```python
from build123d import *

# Parameters (mm, degrees)
SKETCH_1_W              = 20
SKETCH_1_H              = 25
EXTRUDE_1_DEPTH         = 1.5
SKETCH_2_W              = 10.1
SKETCH_2_H              = 17.5
CUT_EXTRUDE_1_DEPTH     = 0.25
HOLE_WIZARD_3_2_3_2_1_D = 3.2
HOLE_WIZARD_3_2_3_2_2_D = 3.2


with BuildPart() as part:
    # 草图1 → 凸台-拉伸1 (new body)
    with BuildSketch(Plane.XZ):
        with Locations((0, -2.5)):
            Rectangle(SKETCH_1_W, SKETCH_1_H)
    extrude(amount=-EXTRUDE_1_DEPTH)

    # 草图2 → 切除-拉伸1 (cut)
    with BuildSketch(Plane.XZ):
        with Locations((0, 1.25)):
            Rectangle(SKETCH_2_W, SKETCH_2_H)
    extrude(amount=-CUT_EXTRUDE_1_DEPTH, mode=Mode.SUBTRACT)

    # Ø3.2 (3.2) 直径孔1 (through all)
    with Locations(Plane(origin=(0, 0, 0), x_dir=(-1, 0, 0), z_dir=(0, -1, 0))):
        with Locations((-7, -7), (-7, 12)):
            Hole(HOLE_WIZARD_3_2_3_2_1_D / 2)

    # Ø3.2 (3.2) 直径孔2 (through all)
    with Locations(Plane(origin=(0, 1.5, 0), x_dir=(1, 0, 0), z_dir=(0, 1, 0))):
        with Locations((-7, -7), (-7, 12)):
            Hole(HOLE_WIZARD_3_2_3_2_2_D / 2)


solid = part.part
```
For this review, take the finished solid that the model builds, in its own axes (mm). A direction names the side the tool comes from. Coordinates: 2 decimals unless noted, no trailing zeros. Loops run counter-clockwise (first coordinate to the right, second up) from the corner with the lowest first, then second, coordinate; pieces in that order, holes last. Notation, with made-up numbers: (47, -40) - (91, -40) arc R25 ccw to (91, -26) - close; hole circle Ø8 at (1.25, -21.75). An arc over 180 degrees is marked (long way). Use one line per item in the form item = value. Start each with the question number.
1) To check wall thickness, follow probe 1 along X at (y, z) = (0.4, 7); probe 2 along Z at (x, y) = (-7, 0.7); probe 3 along Z at (x, y) = (7.5, 0.45). State the ranges of each line that lie inside material, in increasing order. Write a range as from..to.
2) Take a section at B-B (y = 0.8). State the section outline as (x, z) points.
3) Take a section at C-C (x = 7.25). State the section outline as (y, z) points.
4) Take a section at D-D (z = 2.75). State the section outline as (x, y) points.
5) For faces 4 (the face through (0, 1, 10)), 5 (the face through (0, 0.25, 1)), list the 3-axis set-ups (+Z, -Z, +X, -X, +Y, -Y) from which the entire face can be reached by the end or side of a thin tool; tool diameter is ignored.
6) Take a section at A-A (z = -12). State the section outline as (x, y) points.
7) For pin 1 (3 mm diameter, centred on x = -1.5, z = -0.5, fed in from -Y); pin 2 (3 mm diameter, centred on x = 7, z = 7, fed in from +Y); pin 3 (10 mm diameter, centred on x = 4, z = 2.5, fed in from -Y), all flat-tipped, find the tip position at first contact; note any pin that passes through.
8) Draft analysis for pull direction X (two halves, no side actions). For faces 1 (the face through (0, 0, -8)), 2 (the face through (6.65, 0.76, 8.56)), 3 (the face through (10, 1, -3)), state which applies: released by +X, released by -X, zero draft, split by the parting line, or undercut.
From the geometry:
q1.probe_1 = -10..-8.6, -5.4..5.4, 8.6..10
q1.probe_2 = -15..-13.6, -10.4..5.4, 8.6..10
q1.probe_3 = -15..-13.52, -10.48..5.48, 8.52..10
q2.outline = (-10, -15) - (10, -15) - (10, 10) - (-10, 10) - close; hole circle Ø3.2 at (-7, -12); hole circle Ø3.2 at (-7, 7); hole circle Ø3.2 at (7, -12); hole circle Ø3.2 at (7, 7)
q3.outline = (0, -15) - (1.5, -15) - (1.5, -13.58) - (0, -13.58) - close; (0, -10.42) - (1.5, -10.42) - (1.5, 5.42) - (0, 5.42) - close; (0, 8.58) - (1.5, 8.58) - (1.5, 10) - (0, 10) - close
q4.outline = (-10, 0) - (-5.05, 0) - (-5.05, 0.25) - (5.05, 0.25) - (5.05, 0) - (10, 0) - (10, 1.5) - (-10, 1.5) - close
q5.face_4 = +Z, +X, -X, +Y, -Y
q5.face_5 = +Z, -Y
q6.outline = (-10, 0) - (-8.6, 0) - (-8.6, 1.5) - (-10, 1.5) - close; (-5.4, 0) - (5.4, 0) - (5.4, 1.5) - (-5.4, 1.5) - close; (8.6, 0) - (10, 0) - (10, 1.5) - (8.6, 1.5) - close
q7.pin_1 = 0.25
q7.pin_2 = through
q7.pin_3 = 0
q8.face_1 = zero draft
q8.face_2 = undercut
q8.face_3 = released by +X
